from build123d import *

# Parameters (mm, degrees)
SKETCH1_R                = 7
BOSS_EXTRUDE1_DEPTH      = 2.4
BOSS_EXTRUDE3_DEPTH      = 1.55
BOSS_EXTRUDE3_DEPTH_BACK = 1.55


with BuildPart() as part:
    # Sketch1 → Boss-Extrude1 (new body)
    with BuildSketch(Plane(origin=(0, 0, 0), x_dir=(1, 0, 0), z_dir=(0, 1, 0))):
        with Locations(Location((0, 0, 0), (0, 0, 270))):
            Circle(SKETCH1_R)
    extrude(amount=BOSS_EXTRUDE1_DEPTH)

    # Sketch3 → Boss-Extrude3 (add, two sides: drawn at the far end of the back side and taken through both)
    with BuildSketch(Plane.XY.offset(-BOSS_EXTRUDE3_DEPTH_BACK)):
        Polygon((-0.843447487, 2.4), (0, 2.4), (0.856552513, 2.4), (0.856552513, 5.098601719), (2.556552513, 5.098601719), (2.556552513, 7.4), (-2.543447487, 7.4), (-2.543447487, 5.1), (-0.843447487, 5.1), align=None)
    extrude(amount=BOSS_EXTRUDE3_DEPTH + BOSS_EXTRUDE3_DEPTH_BACK)


solid = part.part
Design review of the part built by this model. Coordinates are the model's own, in mm. A direction names the side the tool comes from. Coordinates: 2 decimals unless noted, no trailing zeros. Order: outer loops, then holes, each group sorted by start corner. A loop starts at its lowest first (then second) coordinate and runs counter-clockwise, first axis right, second up.
Item 1: Take a section at D-D, the plane y = 1. Write out the cut boundary in (x, z).
Item 2: Take a section at A-A, the plane z = 0. Write out the cut boundary in (x, y), then the cut area to 3 significant figures.
Item 3: For line 1 (Y direction, x = 3.75, z = 4); line 2 (X direction, y = 5.25, z = 0.5); line 3 (Z direction, x = 0.75, y = 4.5), list the stretches that pass through material, from the lowest coordinate up.
Item 4: Take a section at B-B, the plane x = -2. Write out the cut boundary in (y, z), then the cut area to 3 significant figures.
Item 5: The part is to be moulded in two halves that separate along Y. For faces 6 (the flat face through (-0.843, 4, 0)), 7 (the flat face through (-2, 5.1, 0)), 8 (the flat face through (0, 5, 1.55)), 9 (the flat face through (0, 0, 0)), say which applies: pulls with the +Y half, pulls with the -Y half, needs draft (parallel to the pull), parting line crosses it, or undercut.
Item 6: Take a section at C-C, the plane y = 6.25. Write out the cut boundary in (x, z), then the cut area to 3 significant figures.
Item 7: For faces 1 (the flat face through (0, 5, -1.55)), 2 (the flat face through (2, 5.099, 0)), 3 (the flat face through (-2.543, 6, 0)), 4 (the flat face through (2.557, 6, 0)), 5 (the flat face through (0, 7.4, 0)), list the 3-axis set-ups (+Z, -Z, +X, -X, +Y, -Y) from which the entire face can be reached by the end or side of a thin tool; tool diameter is ignored.
Item 8: For pin 1 Ø0.5 at (x, z) = (1.5, 0.5) entering from -Y; pin 2 Ø1.5 at (x, y) = (0, 4.5) entering from -Z; pin 3 Ø2.5 at (y, z) = (6, -0.5) entering from +X; pin 4 Ø2 at (y, z) = (4, -0.5) entering from +X, all flat-tipped, find the tip position at first contact; note any pin that passes through.
The answers:
1. outline: circle Ø14 at (0, 0)
2. outline: (-7, 0) - (7, 0) - (7, 2.4) - (0.86, 2.4) - (0.86, 5.1) - (2.56, 5.1) - (2.56, 7.4) - (-2.54, 7.4) - (-2.54, 5.1) - (-0.84, 5.1) - (-0.84, 2.4) - (-7, 2.4) - close
2. area: 49.9 mm2
3. line 1: y = 0 to 2.4
3. line 2: x = -2.54 to 2.56
3. line 3: z = -1.55 to 1.55
4. outline: (0, -6.71) - (2.4, -6.71) - (2.4, 6.71) - (0, 6.71) - close; (5.1, -1.55) - (7.4, -1.55) - (7.4, 1.55) - (5.1, 1.55) - close
4. area: 39.3 mm2
5. face 6: undercut
5. face 7: undercut
5. face 8: needs draft
5. face 9: pulls with the -Y half
6. outline: (-2.54, -1.55) - (2.56, -1.55) - (2.56, 1.55) - (-2.54, 1.55) - close
6. area: 15.8 mm2
7. face 1: -Z, +X, -X, +Y
7. face 2: +Z, -Z, +X
7. face 3: +Z, -Z, -X, +Y
7. face 4: +Z, -Z, +X, +Y
7. face 5: +Z, -Z, +X, -X, +Y
8. pin 1: stops at y = 0
8. pin 2: stops at z = -1.55
8. pin 3: stops at x = 2.56
8. pin 4: stops at x = 0.86
